Solid Edge part; units mm, degrees
sketch "Sketch1" plane through (0, 0, 0) normal (0, 0, 1) x (1, 0, 0)
  line L0 (0, 0) -> (-7.62, 0)
  line L1 (-7.62, 0) -> (-7.62, 42.062)
  line L2 (-7.62, 42.062) -> (0, 42.062)
  line L3 (0, 42.062) -> (0, 0)
  dimension "D1" = 7.62
extrude "Protrusion1" add sketch "Sketch1" along normal blind 1.5875
sketch "Sketch2" plane through (-4.1275, 17.6405, 0) normal (0, 0, -1) x (0, 1, 0)
  line L0 (-8.5137, -3.4925) -> (14.2615, -3.4925)
  line L1 (-8.5137, 4.1275) -> (-8.5137, -3.4925)
  line L2 (14.2615, 4.1275) -> (-8.5137, 4.1275)
  line L3 (24.4215, 4.1275) -> (14.2615, 4.1275)
  line L4 (24.4215, -4.1275) -> (24.4215, 4.1275)
  line L5 (14.2615, -4.1275) -> (24.4215, -4.1275)
extrude "Protrusion2" add sketch "Sketch2" along normal up to vertex (1.6684 mm away) material side at (-7.67, 20.5144, 0)
sketch "Sketch3" plane through (-4.1275, 15.951, 0) normal (0, 0, -1) x (-1, 0, 0)
  circle A0 centre (0, 4.1) radius 1.651
extrude "Cutout1" cut sketch "Sketch3" against normal through all and the other way through all
sketch "Sketch4" plane through (-4.1275, 24.3244, -1.6684) normal (0, 0, -1) x (0, 1, 0)
  line L0 (7.6757, 4.1275) -> (13.7987, 4.1275)
  line L1 (13.7987, 4.1275) -> (13.7987, -3.4925)
  line L2 (13.7987, -3.4925) -> (7.6757, -3.4925)
  line L3 (7.6757, -3.4925) -> (7.6757, 4.1275)
extrude "ExtrudedProtrusion_3" add sketch "Sketch4" along normal blind 7.2044
sketch "Sketch5" plane through (-3.81, 21.031, 1.5875) normal (0, 0, 1) x (0, -1, 0)
  line L0 (-4.1, 3.175) -> (-4.1, -3.81)
  line L1 (-4.1, -3.81) -> (6.06, -3.81)
  line L2 (6.06, -3.81) -> (6.06, 3.175)
  line L3 (6.06, 3.81) -> (6.06, 3.175)
  line L4 (-4.1, 3.81) -> (6.06, 3.81)
  line L5 (-4.1, 3.175) -> (-4.1, 3.81)
extrude "ExtrudedProtrusion_4" add sketch "Sketch5" along normal blind 25.1481
sketch "Sketch6" plane through (-4.1275, 20.051, 1.5875) normal (0, 0, -1) x (0, 1, 0)
  circle A0 centre (0, 0) radius 3.105
extrude "Cutout2" cut sketch "Sketch6" against normal through all
CAD build for the part. Positions are in the model's coordinates, mm. A direction names the side the tool comes from. Coordinates: 2 decimals unless noted, no trailing zeros. Write each loop counter-clockwise with the first axis right and the second up, starting at its lowest first coordinate (ties: lowest second). Pieces come first, ordered by that corner, then holes. Notation, with made-up numbers: (40, 72.5) - (84, 72.5) arc R21 cw to (84, 81.5) - close; hole circle Ø10 at (81, 27.25). An arc over 180 degrees is marked (long way). Use a Markdown table: item, result. Add a question column.
Item 1: 3-axis set-ups, long thin cutter, end or side, ignore diameter. For faces 1 (the face through (-4, 5, 0)), 2 (the face through (-4, 34, 1.588)), 3 (the face through (-7.62, 35, -5)), 4 (the face through (-4, 38.123, -5)), 5 (the face through (-4, 14.971, 14)): which of +Z, -Z, +X, -X, +Y, -Y reach the whole face in a straight line?
Item 2: Drill centre lines: L1, parallel to Y at x = -1.5, z = 15; L2, parallel to Z at x = -4.25, y = 11; L3, parallel to Z at x = -0.75, y = 17. Where is each one in solid material? Low to high. Write a range as from..to.
Item 3: Band-saw the part on D-D, the plane z = -1. Give the cut face in (x, y) (1 decimal), and give its area (3 significant figures).
Item 4: Band-saw the part on C-C, the plane x = -3. Give the cut face in (y, z), and give its area (3 significant figures).
Item 5: Band-saw the part on B-B, the plane y = 21. Give the cut face in (x, z), and give its area (3 significant figures).
Item 6: Mould opens along X. For faces 6 (the face through (-5.5, 18.7, 1.588)), 7 (the face through (-0.5, 20.1, 26.736)), 8 (the face through (0, 23, 8)) say: pulls with the +X half, pulls with the -X half, needs draft (parallel to the pull), parting line crosses it, or undercut.
Item 7: Flat gauge pins, fed straight in: pin 1 (2.5 mm diameter, centred on x = -5.5, y = 33, fed in from +Z); pin 2 (1.5 mm diameter, centred on y = 25.5, z = 6, fed in from +X); pin 3 (5 mm diameter, centred on y = 35.5, z = -7, fed in from -X); pin 4 (3.5 mm diameter, centred on x = -4, z = -4.5, fed in from +Y). Where does each tip first touch, or does it go through?
Item 8: Band-saw the part on A-A, the plane x = -0.5. Give the cut face in (y, z), and give its area (3 significant figures).
Numbers:
| question | item | result |
|---|---|---|
| 1 | face 1 | -Z, +X, -X, -Y |
| 1 | face 2 | +Z, +X, -X, +Y |
| 1 | face 3 | -Z, -X, +Y, -Y |
| 1 | face 4 | -Z, +X, -X, +Y |
| 1 | face 5 | +Z, +X, -X, -Y |
| 2 | L1 | 14.97..18.4, 21.71..25.13 |
| 2 | L2 | -1.67..1.59 |
| 2 | L3 | -1.67..26.74 |
| 3 | outline | (-8.3, 31.9) - (-7.6, 31.9) - (-7.6, 9.1) - (0, 9.1) - (0, 42.1) - (-8.3, 42.1) - close; hole circle Ø3.3 at (-4.1, 20.1) |
| 3 | area | 249 mm2 |
| 4 | outline | (0, 0) - (9.13, 0) - (9.13, -1.67) - (18.84, -1.67) - (18.84, 1.59) - (17.16, 1.59) - (17.16, 26.74) - (14.97, 26.74) - (14.97, 1.59) - (0, 1.59) - close; (21.26, -1.67) - (32, -1.67) - (32, -8.87) - (38.12, -8.87) - (38.12, -1.67) - (42.06, -1.67) - (42.06, 1.59) - (25.13, 1.59) - (25.13, 26.74) - (22.94, 26.74) - (22.94, 1.59) - (21.26, 1.59) - close |
| 4 | area | 268 mm2 |
| 5 | outline | (-7.62, -1.67) - (-5.48, -1.67) - (-5.48, 1.59) - (-7.08, 1.59) - (-7.08, 26.74) - (-7.62, 26.74) - close; (-2.78, -1.67) - (0, -1.67) - (0, 26.74) - (-1.17, 26.74) - (-1.17, 1.59) - (-2.78, 1.59) - close |
| 5 | area | 58.9 mm2 |
| 6 | face 6 | undercut |
| 6 | face 7 | needs draft |
| 6 | face 8 | pulls with the +X half |
| 7 | pin 1 | z = 1.59 |
| 7 | pin 2 | x = 0 |
| 7 | pin 3 | x = -7.62 |
| 7 | pin 4 | y = 38.12 |
| 8 | outline | (0, 0) - (9.13, 0) - (9.13, -1.67) - (32, -1.67) - (32, -8.87) - (38.12, -8.87) - (38.12, -1.67) - (42.06, -1.67) - (42.06, 1.59) - (25.13, 1.59) - (25.13, 26.74) - (14.97, 26.74) - (14.97, 1.59) - (0, 1.59) - close |
| 8 | area | 421 mm2 |
